Could you check a few things on this model? Use its own coordinates, in mm. Face numbers are marked on the shaded views. A direction names the side the tool comes from. Round coordinates to 2 decimals unless told otherwise and drop trailing zeros. Write each loop counter-clockwise with the first axis right and the second up, starting at its lowest first coordinate (ties: lowest second). Pieces come first, ordered by that corner, then holes. Notation, with made-up numbers: (10, -1.5) -> (48, -1.5) arc R22 ccw to (48, 24.5) -> close; hole circle Ø8 at (24, 24). An arc over 180 degrees is marked (long way). Return JSON: item names as keys, results as strings.
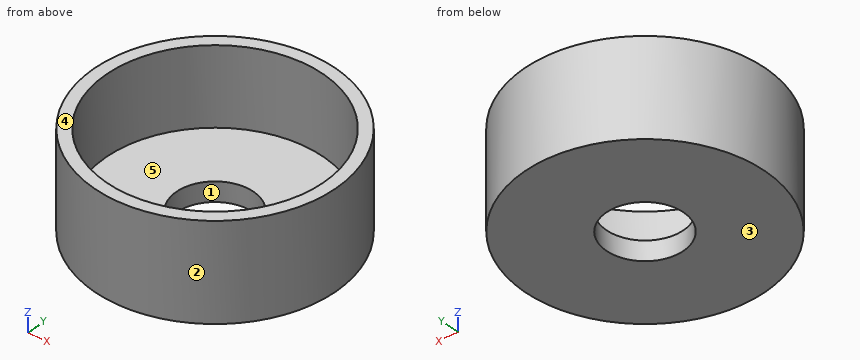
from build123d import *

# Parameters (mm, degrees)
F0_R     = 12.5
F1_DEPTH = 10
F2_R     = 4
F3_DEPTH = 25
F2_R_2   = 11.25
F4_DEPTH = 8


with BuildPart() as f1:
    # F0 (on Top) → F1 (new body)
    with BuildSketch(Plane.XY):
        Circle(F0_R)
    extrude(amount=F1_DEPTH)

    # F2 (on face) → F3 (cut)
    with BuildSketch(Plane.XY.offset(10)):
        Circle(F2_R)
    extrude(amount=-F3_DEPTH, mode=Mode.SUBTRACT)

    # F2 (on face) → F4 (cut)
    with BuildSketch(Plane.XY.offset(10)):
        Circle(F2_R_2)
        Circle(F2_R, mode=Mode.SUBTRACT)
    extrude(amount=-F4_DEPTH, mode=Mode.SUBTRACT)


solid = f1.part
1) I want a section at D-D, the plane y = -5.75. Please give me the cut outline in (x, z), and give its area (3 significant figures).
Return value:
{"outline": "(-11.1, 0) -> (11.1, 0) -> (11.1, 10) -> (9.67, 10) -> (9.67, 2) -> (-9.67, 2) -> (-9.67, 10) -> (-11.1, 10) -> close", "area": "67.3 mm²"}
2) If I drill on probe 1 along Y at (x, z) = (0, 0.45); probe 2 along Y at (x, z) = (0, 5.75); probe 3 along Z at (x, y) = (-7.75, 7), over which ranges is the centre line in solid material (lowest first)? Write a range as [from, to].
Return value:
{"probe 1": "[-12.5, -4], [4, 12.5]", "probe 2": "[-12.5, -11.25], [11.25, 12.5]", "probe 3": "[0, 2]"}
3) I want a section at A-A, the plane x = 0. Please give me the cut outline in (y, z).
Return value:
{"outline": "(-12.5, 0) -> (-4, 0) -> (-4, 2) -> (-11.25, 2) -> (-11.25, 10) -> (-12.5, 10) -> close; (4, 0) -> (12.5, 0) -> (12.5, 10) -> (11.25, 10) -> (11.25, 2) -> (4, 2) -> close"}
4) I want a section at C-C, the plane z = 4. Please give me the cut outline in (x, y).
Return value:
{"outline": "circle Ø25 at (0, 0); hole circle Ø22.5 at (0, 0)"}
5) For the marked faces 4 and 5, which set-ups out of +Z, -Z, +X, -X, +Y, -Y let a thin tool reach every point of the face, with its end or its side?
Return value:
{"face 4": "+Z, +X, -X, +Y, -Y", "face 5": "+Z"}
6) Thinking about a two-plate mould opening in Y: for the marked faces 1, 2 and 3, which applies, pulls with the +Y half, pulls with the -Y half, needs draft (parallel to the pull), parting line crosses it, or undercut?
Return value:
{"face 1": "undercut", "face 2": "parting line crosses it", "face 3": "needs draft"}
7) Will these pins go through, and if not, where does the flat tip stop? pin 1 Ø5 at (y, z) = (-4.5, 4) entering from -X; pin 2 Ø1.5 at (x, y) = (-9.5, 4) entering from +Z; pin 3 Ø3 at (x, z) = (-7.5, 6.5) entering from -Y.
Return value:
{"pin 1": "x = -12.34", "pin 2": "z = 2", "pin 3": "y = -10.97"}
